Study the drawing (mm; zero at the part's minimum x, y, z) and answer. A direction names the side the tool comes from. Give positions to 0.01 mm unless a question says otherwise; leave off trailing zeros. Write each loop counter-clockwise with the first axis right and the second up, starting at its lowest first coordinate (ties: lowest second). Pieces come first, ordered by that corner, then holes. Notation, with made-up numbers: M 75.25,1.25 L 100.25,1.25 A17 ccw 100.25,6.25 Z; hole C 70.5,-10 d7. An arc over 180 degrees is marked long. Use a Markdown table: item, result. Add a question column.
Item 1: Consider probe 1 along X at (y, z) = (76.2, 18.5) (3 decimals); probe 2 along Z at (x, y) = (126.5, 52); probe 3 along X at (y, z) = (139, 52). Determine where each line is inside the solid, lowest interval first. Write a range as [from, to].
Item 2: A cutting plane is placed at B-B on x = 39.5. Determine the outline of the cut face in (y, z) (3 decimals).
Item 3: Given P1, Ø10, axis at y = 43.5, z = 45.5, coming from the -X side; P2, Ø2.5, axis at x = 33, z = 54, coming from the +Y side; P3, Ø4, axis at y = 44.5, z = 50, coming from the -X side, each flat-ended and moving along its own axis, determine where each tip first touches the part or whether it passes through.
Item 4: For the marked faces 1, 2 and 3, determine the directions among +Z, -Z, +X, -X, +Y, -Y from which every point of the face is accessible in a straight line to the end or side of a thin tool.
Item 5: A cutting plane is placed at C-C on y = 12.7. Determine the outline of the cut face in (x, z) (3 decimals).
Item 6: A cutting plane is placed at A-A on z = 50.5. Determine the outline of the cut face in (x, y) (3 decimals), then the cut area to 3 significant figures.
Item 7: A cutting plane is placed at D-D on z = 16. Determine the outline of the cut face in (x, y) (3 decimals).
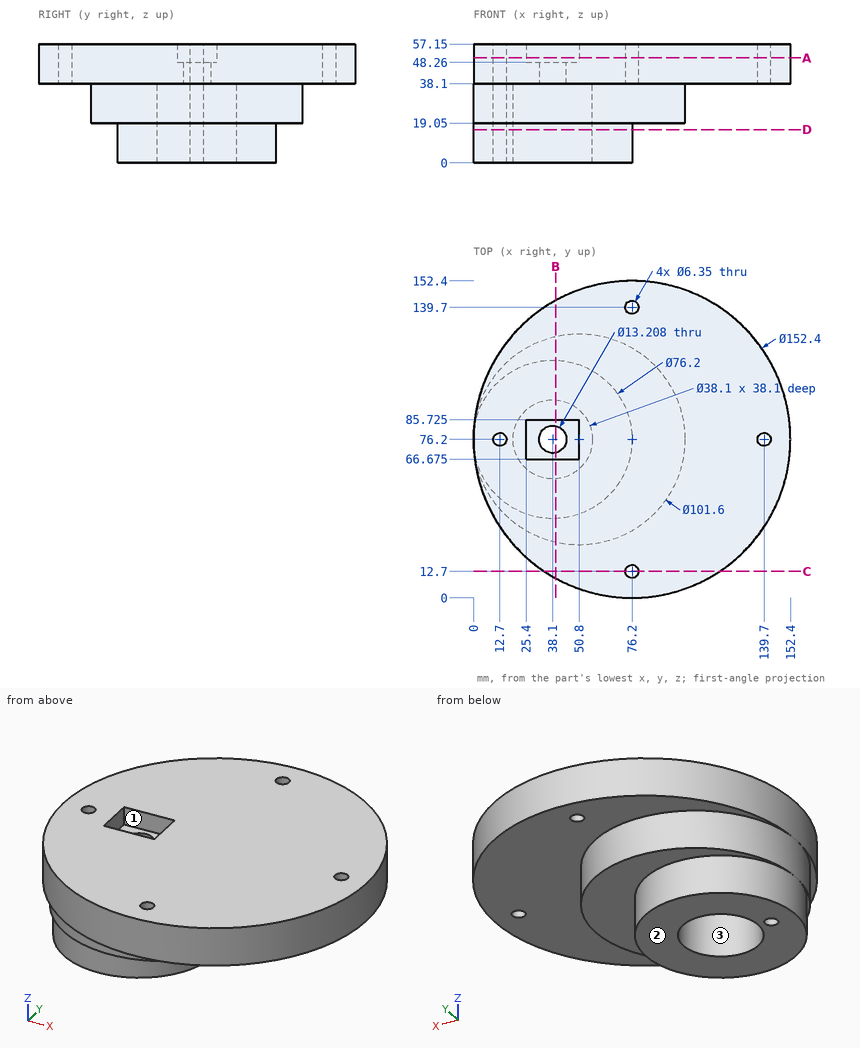
Filled in:
| question | item | result |
|---|---|---|
| 1 | probe 1 | [0, 9.525], [15.875, 19.05], [57.15, 76.2] |
| 1 | probe 2 | [38.1, 57.15] |
| 1 | probe 3 | [33.04, 73.1], [79.3, 119.36] |
| 2 | outline | M 9.42,38.1 L 26.673,38.1 L 26.673,19.05 L 38.126,19.05 L 38.126,0 L 57.202,0 L 57.202,38.1 L 69.746,38.1 L 69.746,48.26 L 66.675,48.26 L 66.675,57.15 L 9.42,57.15 Z; M 82.654,38.1 L 95.198,38.1 L 95.198,0 L 114.274,0 L 114.274,19.05 L 125.727,19.05 L 125.727,38.1 L 142.98,38.1 L 142.98,57.15 L 85.725,57.15 L 85.725,48.26 L 82.654,48.26 Z |
| 3 | P1 | x = 5.21 |
| 3 | P2 | y = 139.81 |
| 3 | P3 | x = 6.03 |
| 4 | face 1 | +Z |
| 4 | face 2 | -Z, +X, -X, +Y, -Y |
| 4 | face 3 | -Z |
| 5 | outline | M 34.079,38.1 L 73.025,38.1 L 73.025,57.15 L 34.079,57.15 Z; M 79.375,38.1 L 118.321,38.1 L 118.321,57.15 L 79.375,57.15 Z |
| 6 | outline | C 76.2,76.2 d152.4; hole C 12.7,76.2 d6.35; hole M 25.4,66.675 L 50.8,66.675 L 50.8,85.725 L 25.4,85.725 Z; hole C 76.2,12.7 d6.35; hole C 76.2,139.7 d6.35; hole C 139.7,76.2 d6.35 |
| 6 | area | 17,600 mm² |
| 7 | outline | C 38.1,76.2 d76.2; hole C 12.7,76.2 d6.35; hole C 38.1,76.2 d38.1 |
